For this review, use the dimensioned drawing (mm, ordinates from the lowest corner) and the shaded views. Coordinates: 2 decimals unless noted, no trailing zeros. Write each loop counter-clockwise with the first axis right and the second up, starting at its lowest first coordinate (ties: lowest second). Pieces come first, ordered by that corner, then holes. Notation, with made-up numbers: (81, -23.5) -> (134, -23.5) arc R28 cw to (134, 3.5) -> close; hole circle Ø4 at (7.25, -18.5). An arc over 180 degrees is marked (long way). Put each result on its own line as item: value. Start each with the question number.
Item 1: Consider section A-A on z = 1.15. Give the boundary of the cut face in (x, y) (1 decimal), and give its area (3 significant figures).
Item 2: Consider section B-B on y = 1.55. Give the number of separate pieces and of enclosed holes in the cut face, and give its area (3 significant figures).
Item 3: To check wall thickness, follow L1, parallel to X at y = 2.35, z = 3.4 (1 decimal); L2, parallel to Y at x = 2.5, z = 2.75; L3, parallel to X at y = 2.2, z = 2.5 (1 decimal). State the ranges of each line that lie inside material, in increasing order.
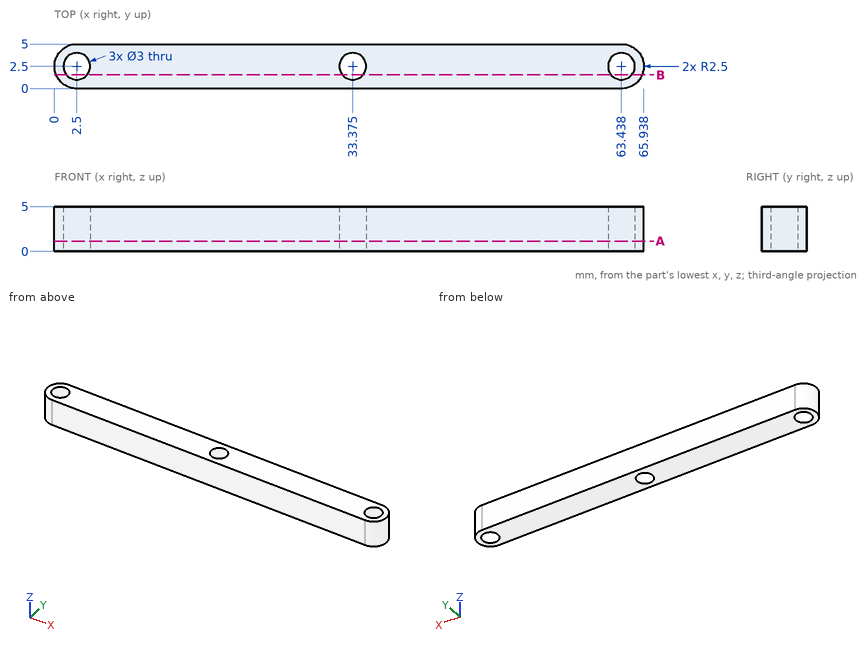
Return value:
1. outline: (2.5, 0) -> (63.4, 0) arc R2.5 ccw to (63.4, 5) -> (2.5, 5) arc R2.5 ccw to start; hole circle Ø3 at (2.5, 2.5); hole circle Ø3 at (33.4, 2.5); hole circle Ø3 at (63.4, 2.5)
1. area: 303 mm^2
2. separate pieces: 4
2. enclosed holes: 0
2. area: 293 mm^2
3. L1: 0 to 1, 4 to 31.9, 34.9 to 61.9, 64.9 to 65.9
3. L2: 0 to 1, 4 to 5
3. L3: 0 to 1, 4 to 31.9, 34.8 to 62, 64.9 to 65.9
